Design review of the part built by this model. Coordinates are the model's own, in mm. Round coordinates to 2 decimals unless told otherwise and drop trailing zeros. Order: outer loops, then holes, each group sorted by start corner. A loop starts at its lowest first (then second) coordinate and runs counter-clockwise, first axis right, second up.
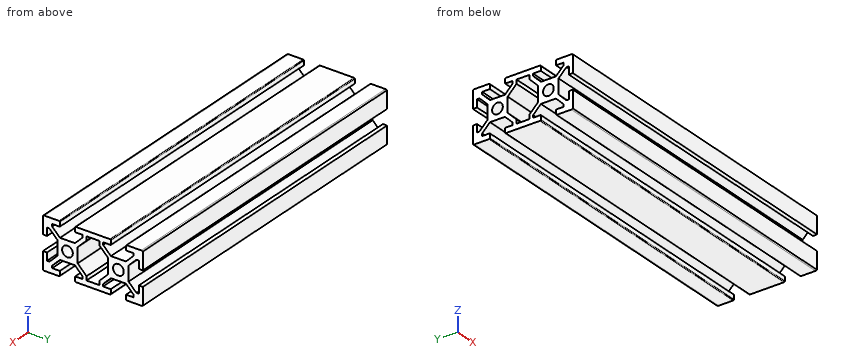
from build123d import *

# Parameters (mm, degrees)
SKETCH_1_R                   = 2.1
SERI_5_20_40_20X40S5_2_DEPTH = 130


with BuildPart() as part:
    # 草图1 → Seri 5 (20,40) 20X40S5(2) (new body)
    with BuildSketch(Plane(origin=(0, 0, 0), x_dir=(0, 0, -1), z_dir=(1, 0, 0))):
        with BuildLine():
            Line((-10, 19), (-10, 13.3))
            ThreePointArc((-10, 13.3), (-9.912132034, 13.087867966), (-9.7, 13))
            Line((-9.7, 13), (-8, 13))
            Line((-8, 13), (-8, 16))
            Line((-8, 16), (-7.060660172, 16))
            Line((-7.060660172, 16), (-4, 12.939339828))
            Line((-4, 12.939339828), (-4, 7.060660172))
            Line((-4, 7.060660172), (-7.060660172, 4))
            Line((-7.060660172, 4), (-8, 4))
            Line((-8, 4), (-8, 7))
            Line((-8, 7), (-9.7, 7))
            ThreePointArc((-9.7, 7), (-9.912132034, 6.912132034), (-10, 6.7))
            Line((-10, 6.7), (-10, -6.7))
            ThreePointArc((-10, -6.7), (-9.912132034, -6.912132034), (-9.7, -7))
            Line((-9.7, -7), (-8, -7))
            Line((-8, -7), (-8, -4))
            Line((-8, -4), (-7.060660172, -4))
            Line((-7.060660172, -4), (-4, -7.060660172))
            Line((-4, -7.060660172), (-4, -12.939339828))
            Line((-4, -12.939339828), (-7.060660172, -16))
            Line((-7.060660172, -16), (-8, -16))
            Line((-8, -16), (-8, -13))
            Line((-8, -13), (-9.7, -13))
            ThreePointArc((-9.7, -13), (-9.912132034, -13.087867966), (-10, -13.3))
            Line((-10, -13.3), (-10, -19))
            ThreePointArc((-10, -19), (-9.948683298, -19.316227766), (-9.8, -19.6))
            Line((-9.8, -19.6), (-3, -19.6))
            Line((-3, -19.6), (-3, -18))
            Line((-3, -18), (-6, -18))
            Line((-6, -18), (-6, -17.060660172))
            Line((-6, -17.060660172), (-2.939339828, -14))
            Line((-2.939339828, -14), (2.939339828, -14))
            Line((2.939339828, -14), (6, -17.060660172))
            Line((6, -17.060660172), (6, -18))
            Line((6, -18), (3, -18))
            Line((3, -18), (3, -19.6))
            Line((3, -19.6), (9.8, -19.6))
            ThreePointArc((9.8, -19.6), (9.948683298, -19.316227766), (10, -19))
            Line((10, -19), (10, -13.3))
            ThreePointArc((10, -13.3), (9.912132034, -13.087867966), (9.7, -13))
            Line((9.7, -13), (8, -13))
            Line((8, -13), (8, -16))
            Line((8, -16), (7.060660172, -16))
            Line((7.060660172, -16), (4, -12.939339828))
            Line((4, -12.939339828), (4, -7.060660172))
            Line((4, -7.060660172), (7.060660172, -4))
            Line((7.060660172, -4), (8, -4))
            Line((8, -4), (8, -7))
            Line((8, -7), (9.7, -7))
            ThreePointArc((9.7, -7), (9.912132034, -6.912132034), (10, -6.7))
            Line((10, -6.7), (10, 6.7))
            ThreePointArc((10, 6.7), (9.912132034, 6.912132034), (9.7, 7))
            Line((9.7, 7), (8, 7))
            Line((8, 7), (8, 4))
            Line((8, 4), (7.060660172, 4))
            Line((7.060660172, 4), (4, 7.060660172))
            Line((4, 7.060660172), (4, 12.939339828))
            Line((4, 12.939339828), (7.060660172, 16))
            Line((7.060660172, 16), (8, 16))
            Line((8, 16), (8, 13))
            Line((8, 13), (9.7, 13))
            ThreePointArc((9.7, 13), (9.912132034, 13.087867966), (10, 13.3))
            Line((10, 13.3), (10, 19))
            ThreePointArc((10, 19), (9.948683298, 19.316227766), (9.8, 19.6))
            Line((9.8, 19.6), (3, 19.6))
            Line((3, 19.6), (3, 18))
            Line((3, 18), (6, 18))
            Line((6, 18), (6, 17.060660172))
            Line((6, 17.060660172), (2.939339828, 14))
            Line((2.939339828, 14), (-2.939339828, 14))
            Line((-2.939339828, 14), (-6, 17.060660172))
            Line((-6, 17.060660172), (-6, 18))
            Line((-6, 18), (-3, 18))
            Line((-3, 18), (-3, 19.6))
            Line((-3, 19.6), (-9.8, 19.6))
            ThreePointArc((-9.8, 19.6), (-9.948683298, 19.316227766), (-10, 19))
        make_face()
        with Locations((0, -10)):
            Circle(SKETCH_1_R, mode=Mode.SUBTRACT)
        with Locations((0, 10)):
            Circle(SKETCH_1_R, mode=Mode.SUBTRACT)
        Polygon((-8, -2.5), (-6.439339828, -2.5), (-2.939339828, -6), (2.939339828, -6), (6.439339828, -2.5), (8, -2.5), (8, 2.5), (6.439339828, 2.5), (2.939339828, 6), (-2.939339828, 6), (-6.439339828, 2.5), (-8, 2.5), align=None, mode=Mode.SUBTRACT)
    extrude(amount=SERI_5_20_40_20X40S5_2_DEPTH)


solid = part.part
1) To check wall thickness, follow line 1 along Y through (x, z) = (30, 0); line 2 along Z through (x, y) = (122.5, -1); line 3 along Y through (x, z) = (36.5, -4.75). State the ranges of each line that lie inside material, in increasing order.
Results:
line 1: y = -14 to -12.1, -7.9 to -6, 6 to 7.9, 12.1 to 14
line 2: z = -10 to -8, 8 to 10
line 3: y = -19.6 to -18, -15.81 to -13.69, -6.31 to -4.19, 4.19 to 6.31, 13.69 to 15.81, 18 to 19.6
2) Clearance check with flat-ended pins moving along their axes: P1, Ø5, axis at y = 1, z = 5, coming from the +X side; P2, Ø1.5, axis at x = 116.5, y = 8.5, coming from the +Z side; P3, Ø2, axis at x = 21.5, z = -0.5, coming from the +Y side. State where each tip first meets the part, or that it passes through.
Results:
P1: stops at x = 130
P2: stops at z = 4
P3: stops at y = 14
3) Take a section at A-A on y = 10. Give the boundary of the cut face in (x, z), plus the area to 3 significant figures.
Results:
outline: (0, -4) - (130, -4) - (130, -2.1) - (0, -2.1) - close; (0, 2.1) - (130, 2.1) - (130, 4) - (0, 4) - close
area: 494 mm2
4) Take a section at C-C on x = 67. State how many separate pieces and enclosed holes the cut face has, plus the area to 3 significant figures.
Results:
separate pieces: 1
enclosed holes: 3
area: 311 mm2
5) Take a section at B-B on z = 0. Give the boundary of the cut face in (x, y).
Results:
outline: (0, -14) - (130, -14) - (130, -12.1) - (0, -12.1) - close; (0, -7.9) - (130, -7.9) - (130, -6) - (0, -6) - close; (0, 6) - (130, 6) - (130, 7.9) - (0, 7.9) - close; (0, 12.1) - (130, 12.1) - (130, 14) - (0, 14) - close
